The drawing under review shows one solid part. Ordinate dimensions are in mm from its lowest x, y, z. A direction names the side the tool comes from. Coordinates: 2 decimals unless noted, no trailing zeros. Order: outer loops, then holes, each group sorted by start corner. A loop starts at its lowest first (then second) coordinate and runs counter-clockwise, first axis right, second up. Notation, with made-up numbers: (74.5, 30.5) -> (132.5, 30.5) arc R18 ccw to (132.5, 64.5) -> close; hole circle Ø6 at (32.5, 47). An arc over 180 degrees is marked (long way). Use one line per item in the form item = value.
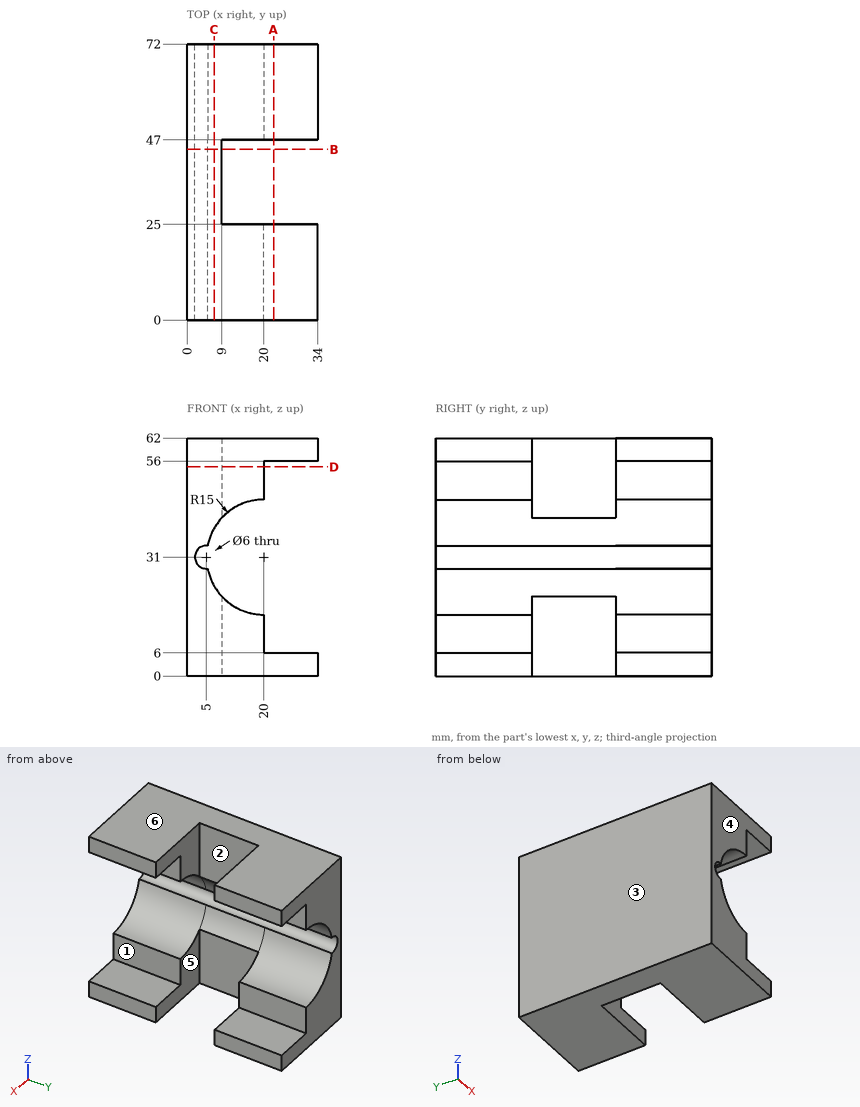
Item 1: We need section D-D (z = 54.5). Write out the cut boundary in (x, y), plus the area to 3 significant figures.
Results found:
outline = (0, 0) -> (20, 0) -> (20, 25) -> (9, 25) -> (9, 47) -> (20, 47) -> (20, 72) -> (0, 72) -> close
area = 1,200 mm²
Item 2: Tool access review of the marked faces 1, 2 and 3: name each direction out of +Z, -Z, +X, -X, +Y, -Y from which nothing blocks a thin tool from reaching the whole face with its end or side.
Results found:
face_1 = +X, +Y, -Y
face_2 = +Z, -Z, +X
face_3 = +Z, -Z, -X, +Y, -Y
Item 3: Clearance check with flat-ended pins moving along their axes: pin 1 (8 mm diameter, centred on y = 6.5, z = 11.5, fed in from +X); pin 2 (10.5 mm diameter, centred on y = 32.5, z = 8, fed in from +X); pin 3 (10 mm diameter, centred on y = 19, z = 28.5, fed in from +X). State where each tip first meets the part, or that it passes through.
Results found:
pin_1 = 20
pin_2 = 9
pin_3 = 7.01
Item 4: We need section C-C (x = 7). Write out the cut boundary in (y, z), plus the area to 3 significant figures.
Results found:
outline = (0, 0) -> (72, 0) -> (72, 23.52) -> (0, 23.52) -> close; (0, 38.48) -> (72, 38.48) -> (72, 62) -> (0, 62) -> close
area = 3,390 mm²
Item 5: Draft analysis for pull direction Y (two halves, no side actions). For the marked faces 4, 5 and 6, state which applies: released by +Y, released by -Y, zero draft, split by the parting line, or undercut.
Results found:
face_4 = released by -Y
face_5 = undercut
face_6 = zero draft
Item 6: We need section B-B (y = 44.5). Write out the cut boundary in (x, z).
Results found:
outline = (0, 0) -> (9, 0) -> (9, 20.8) arc R15 cw to (5.3, 28.02) arc R3 cw (long way) to (5.3, 33.98) arc R15 cw to (9, 41.2) -> (9, 62) -> (0, 62) -> close
Item 7: We need section A-A (x = 22.5). Write out the cut boundary in (y, z).
Results found:
outline = (0, 0) -> (25, 0) -> (25, 6) -> (0, 6) -> close; (0, 56) -> (25, 56) -> (25, 62) -> (0, 62) -> close; (47, 0) -> (72, 0) -> (72, 6) -> (47, 6) -> close; (47, 56) -> (72, 56) -> (72, 62) -> (47, 62) -> close
Item 8: To check wall thickness, follow L1, parallel to Z at x = 5, y = 32; L2, parallel to X at y = 45, z = 53; L3, parallel to Y at x = 11, z = 6. State the ranges of each line that lie inside material, in increasing order. Write a range as from..to.
Results found:
L1 = 0..28, 34..62
L2 = 0..9
L3 = 0..25, 47..72
